Geometry check sheet. Reference: drawing and pictorial views, mm from the part's lowest x, y, z. A direction names the side the tool comes from. Give positions to 0.01 mm unless a question says otherwise; leave off trailing zeros. Write each loop counter-clockwise with the first axis right and the second up, starting at its lowest first coordinate (ties: lowest second). Pieces come first, ordered by that corner, then holes.
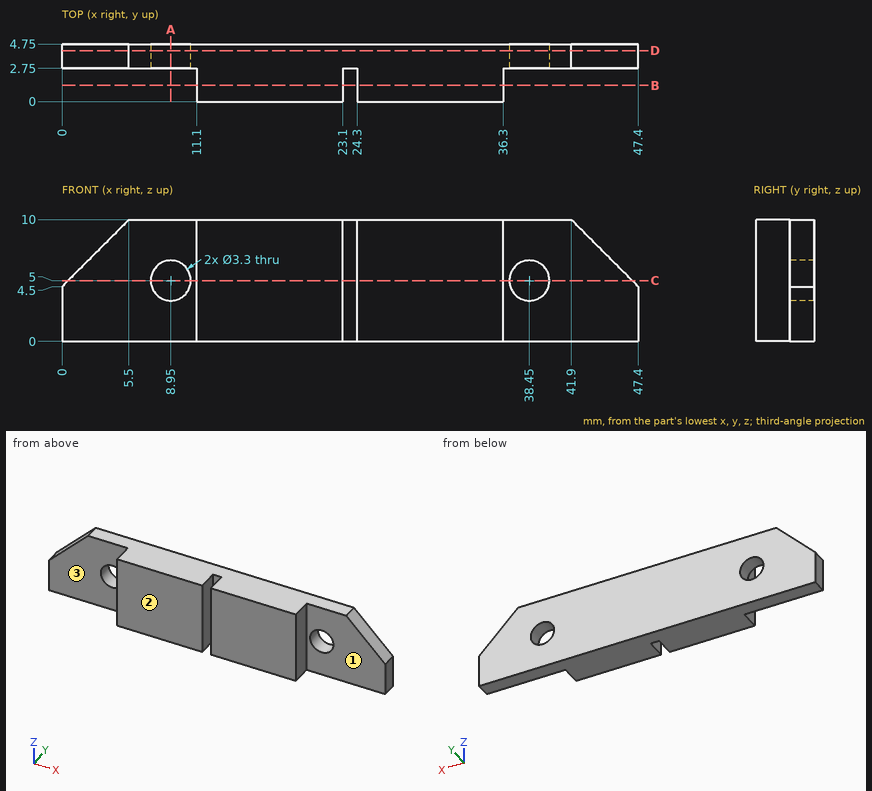
Item 1: Sectioned sample at A-A on x = 8.95. Record the cut outline in (y, z), then the cut area to 3 significant figures.
Answer key:
outline: (2.75, 0) - (4.75, 0) - (4.75, 3.35) - (2.75, 3.35) - close; (2.75, 6.65) - (4.75, 6.65) - (4.75, 10) - (2.75, 10) - close
area: 13.4 mm2
Item 2: Set-up check for the marked faces 1, 2 and 3: record each of +Z, -Z, +X, -X, +Y, -Y from which the full face is reachable in a straight line by a thin tool's end or side.
Answer key:
face 1: +Z, -Z, +X, -Y
face 2: +Z, -Z, +X, -X, -Y
face 3: +Z, -Z, -X, -Y
Item 3: Scan lines: line 1 along Z through (x, y) = (38.45, 3.9); line 2 along X through (y, z) = (1, 9.75); line 3 along Y through (x, z) = (7, 5.25). Record each from-to range of solid material in increasing order.
Answer key:
line 1: z = 0 to 3.35, 6.65 to 10
line 2: x = 11.1 to 23.1, 24.3 to 36.3
line 3: y = 2.75 to 4.75
Item 4: Depth check by flat-ended pin: pin 1 (2 mm diameter, centred on y = 1.5, z = 3, fed in from -X); pin 2 (3 mm diameter, centred on x = 44, z = 6.5, fed in from -Y); pin 3 (0.8 mm diameter, centred on y = 2, z = 7, fed in from +X). Enter the tip coordinate at first touch or a pass-through.
Answer key:
pin 1: stops at x = 11.1
pin 2: stops at y = 2.75
pin 3: stops at x = 36.3
Item 5: Sectioned sample at C-C on z = 5. Record the cut outline in (x, y).
Answer key:
outline: (0.5, 2.75) - (7.3, 2.75) - (7.3, 4.75) - (0.5, 4.75) - close; (10.6, 2.75) - (11.1, 2.75) - (11.1, 0) - (23.1, 0) - (23.1, 2.75) - (24.3, 2.75) - (24.3, 0) - (36.3, 0) - (36.3, 2.75) - (36.8, 2.75) - (36.8, 4.75) - (10.6, 4.75) - close; (40.1, 2.75) - (46.9, 2.75) - (46.9, 4.75) - (40.1, 4.75) - close
Item 6: Sectioned sample at B-B on y = 1.35. Record the cut outline in (x, z).
Answer key:
outline: (11.1, 0) - (23.1, 0) - (23.1, 10) - (11.1, 10) - close; (24.3, 0) - (36.3, 0) - (36.3, 10) - (24.3, 10) - close
Item 7: Sectioned sample at D-D on y = 4.2. Record the cut outline in (x, z), then the cut area to 3 significant figures.
Answer key:
outline: (0, 0) - (47.4, 0) - (47.4, 4.5) - (41.9, 10) - (5.5, 10) - (0, 4.5) - close; hole circle Ø3.3 at (8.95, 5); hole circle Ø3.3 at (38.45, 5)
area: 427 mm2
